Geometry: final body of the model. Coordinates: model frame, mm. Give positions to 0.01 mm unless a question says otherwise; leave off trailing zeros. Order: outer loops, then holes, each group sorted by start corner. A loop starts at its lowest first (then second) coordinate and runs counter-clockwise, first axis right, second up. Notation, with made-up numbers: (78, -30.75) -> (118, -30.75) arc R30 cw to (118, -6.75) -> close; hole circle Ø5 at (32.5, 82). An arc over 180 degrees is marked (long way). One line per item, written item: value. Start each with the question number.
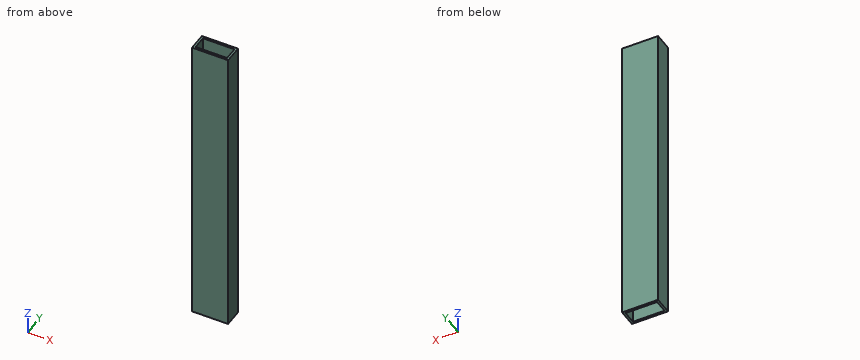
Autodesk Inventor part; units mm, degrees
ref_plane "Start Plane" through (0, 0, 12.7) normal (0, 0, 1) x (1, 0, 0)
ref_plane "End Plane" through (0, 0, 438.15) normal (0, 0, 1) x (1, 0, 0)
ref_plane "Work Plane5" through (25.4, 419.1, 12.7) normal (0, 0, -1) x (-1, 0, 0)
ref_plane "Start Plane" through (0, 0, 12.7) normal (0, 0, 1) x (1, 0, 0)
ref_plane "End Plane" through (0, 0, 438.15) normal (0, 0, 1) x (1, 0, 0)
sketch "Sketch" plane through (0, 0, 0) normal (0, 0, 1) x (1, 0, 0)
  line L0 (-25.4, -12.7) -> (25.4, -12.7)
  line L1 (25.4, -12.7) -> (25.4, 12.7)
  line L2 (25.4, 12.7) -> (-25.4, 12.7)
  line L3 (-25.4, 12.7) -> (-25.4, -12.7)
  line L4 (-25.4, -12.7) -> (25.4, 12.7) construction
  line L5 (25.4, -12.7) -> (-25.4, 12.7) construction
  line L6 (-22.225, -9.525) -> (22.225, -9.525)
  line L7 (22.225, -9.525) -> (22.225, 9.525)
  line L8 (22.225, 9.525) -> (-22.225, 9.525)
  line L9 (-22.225, 9.525) -> (-22.225, -9.525)
  line L10 (-22.225, -9.525) -> (22.225, 9.525) construction
  line L11 (22.225, -9.525) -> (-22.225, 9.525) construction
  point P0 (0, 0)
  point P1 (0, 0)
  dimension "d0" = 50.8
  dimension "d1" = 25.4
  dimension "d2" = 3.175
  dimension "d3" = 3.175
extrude "Body" add sketch "Sketch" along normal up to surface (425.45 mm away) from surface at 12.7
sketch "Sketch4" plane through (0, 0, 0) normal (0, 0, 1) x (1, 0, 0)
  line L0 (0, 0) -> (10, 0)
ref_plane "Work Plane4" through (0, 0, 0) normal (0, -1, 0) x (1, 0, 0)
sketch "Sketch5" plane through (0, 0, 0) normal (0, -1, 0) x (1, 0, 0)
  line L0 (-2, 12.7) -> (12, 12.7)
  line L1 (-2, 438.15) -> (12, 438.15)
  dimension "d11" = 425.45
ref_plane "Work Plane5" through (25.4, 419.1, 12.7) normal (0, 0, -1) x (-1, 0, 0)
split "Split1" plane through (25.4, 419.1, 12.7) removes the side toward (0, 0, -1)
ref_plane "Work Plane6" through (25.4, -203.2, 438.15) normal (0, 0, 1) x (1, 0, 0)
split "Split2" plane through (25.4, -203.2, 438.15) removes the side toward (0, 0, 1)
equation "\"G_OFFSET_START\" = -12.7"
equation "\"G_OFFSET_END\" = -12.7"
equation "\"d6\" = -G_OFFSET_START"
equation "\"d7\" = length + G_OFFSET_END"
equation "\"G_L\" = d11"
properties part number "2x1inTubing"
1. Cut plane C-C, the plane y = 0.25. Return loops of the section in (x, z) (3 decimals), then the cut area to 3 significant figures.
2. Cut plane B-B, the plane x = 9. Return loops of the section in (y, z) (3 decimals).
3. Cut plane A-A, the plane z = 138. Return loops of the section in (x, y) (3 decimals).
4. Material intervals for L1, parallel to Y at x = 9, z = 243.5 (3 decimals); L2, parallel to X at y = -2.25, z = 361 (3 decimals), sorted ascending. Write a range as [from, to].
Answers follow:
1. outline: (-25.4, 12.7) -> (-22.225, 12.7) -> (-22.225, 438.15) -> (-25.4, 438.15) -> close; (22.225, 12.7) -> (25.4, 12.7) -> (25.4, 438.15) -> (22.225, 438.15) -> close
1. area: 2,700 mm²
2. outline: (-12.7, 12.7) -> (-9.525, 12.7) -> (-9.525, 438.15) -> (-12.7, 438.15) -> close; (9.525, 12.7) -> (12.7, 12.7) -> (12.7, 438.15) -> (9.525, 438.15) -> close
3. outline: (-25.4, -12.7) -> (25.4, -12.7) -> (25.4, 12.7) -> (-25.4, 12.7) -> close; hole (-22.225, -9.525) -> (22.225, -9.525) -> (22.225, 9.525) -> (-22.225, 9.525) -> close
4. L1: y = [-12.7, -9.525], [9.525, 12.7]
4. L2: x = [-25.4, -22.225], [22.225, 25.4]
